Can you work these out from the drawing? Everything is in mm from the part's minimum corner. A direction names the side the tool comes from. Give positions to 0.01 mm unless a question says otherwise; leave off trailing zeros. Write each loop counter-clockwise with the first axis right and the second up, starting at its lowest first coordinate (ties: lowest second). Pieces come first, ordered by that corner, then holes. Notation, with made-up numbers: (61, 22) - (116, 22) arc R22 cw to (116, 54) - close; hole circle Ø9 at (26.5, 62.25). An arc over 180 degrees is marked (long way). Answer in a Markdown table with one row per item.
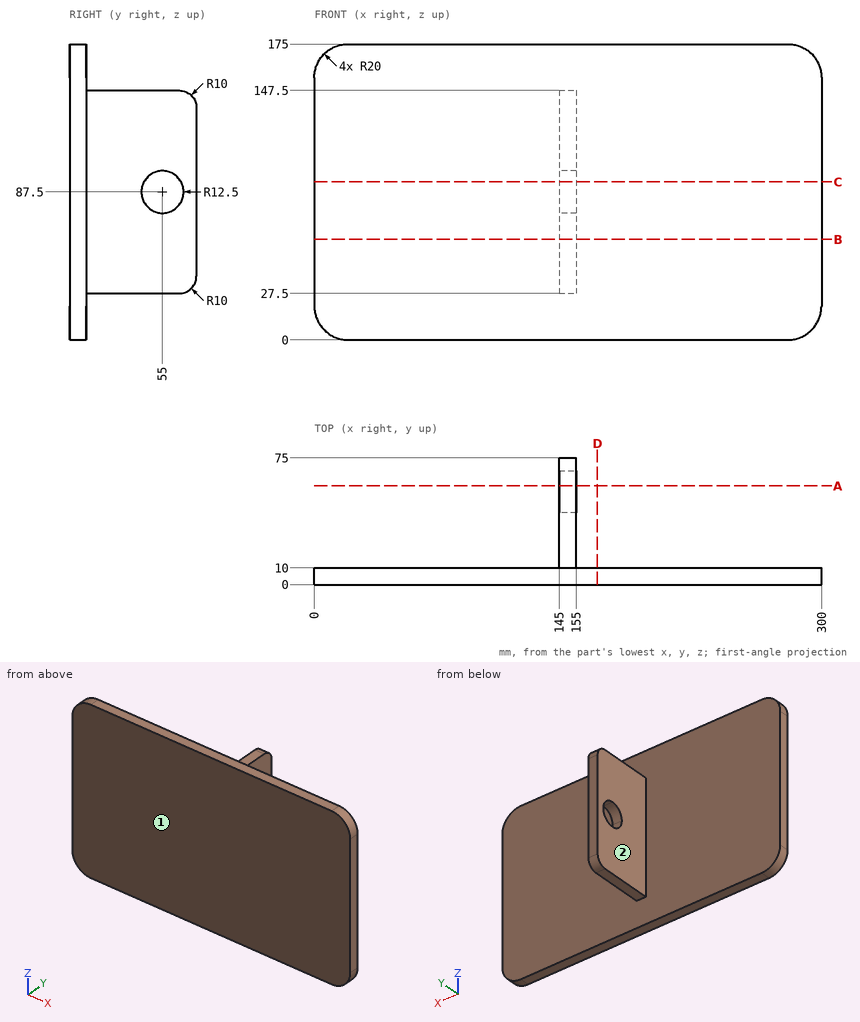
1) If I drill on line 1 (X direction, y = 38, z = 118.5); line 2 (Y direction, x = 149.5, z = 149); line 3 (Z direction, x = 145.5, y = 58), over which ranges is the centre line in solid material (lowest first)?
Check values:
| item | result |
|---|---|
| line 1 | x = 145 to 155 |
| line 2 | y = 0 to 10 |
| line 3 | z = 27.5 to 75.37, 99.63 to 147.5 |
2) Imagine slicing it at C-C (z = 93.5). List the corners of the cut face in (x, y) for me, then the cut area to 3 significant figures.
Check values:
| item | result |
|---|---|
| outline | (0, 0) - (300, 0) - (300, 10) - (155, 10) - (155, 44.03) - (145, 44.03) - (145, 10) - (0, 10) - close; (145, 65.97) - (155, 65.97) - (155, 75) - (145, 75) - close |
| area | 3,430 mm2 |
3) On a 3-axis mill with a long thin cutter (end or side, diameter ignored), from which of +Z, -Z, +X, -X, +Y, -Y can I reach the whole of each face in a straight line? I mean the marked faces 1 and 2. Say none if no direction works.
Check values:
| item | result |
|---|---|
| face 1 | +Z, -Z, +X, -X, -Y |
| face 2 | +Z, -Z, -X, +Y |
4) Imagine slicing it at B-B (z = 59.5). List the corners of the cut face in (x, y) for me.
Check values:
| item | result |
|---|---|
| outline | (0, 0) - (300, 0) - (300, 10) - (155, 10) - (155, 75) - (145, 75) - (145, 10) - (0, 10) - close |
5) Will these pins go through, and if not, where does the flat tip stop? P1, Ø4, axis at x = 136, z = 72.5, coming from the +Y side; P2, Ø12, axis at y = 43, z = 77, coming from the +X side; P3, Ø8, axis at x = 148.5, y = 27, coming from the +Z side; P4, Ø12, axis at x = 174.5, z = 49, coming from the -Y side.
Check values:
| item | result |
|---|---|
| P1 | stops at y = 10 |
| P2 | stops at x = 155 |
| P3 | stops at z = 147.5 |
| P4 | stops at y = 0 |
6) Imagine slicing it at A-A (y = 58.5). List the corners of the cut face in (x, z) for me, then the cut area to 3 significant figures.
Check values:
| item | result |
|---|---|
| outline | (145, 27.5) - (155, 27.5) - (155, 75.5) - (145, 75.5) - close; (145, 99.5) - (155, 99.5) - (155, 147.5) - (145, 147.5) - close |
| area | 960 mm2 |
7) Imagine slicing it at D-D (x = 167.5). List the corners of the cut face in (y, z) for me, then the cut area to 3 significant figures.
Check values:
| item | result |
|---|---|
| outline | (0, 0) - (10, 0) - (10, 175) - (0, 175) - close |
| area | 1,750 mm2 |
